Here's how the part is built. I have some questions about the finished solid (model axes, mm). A direction names the side the tool comes from. Round coordinates to 2 decimals unless told otherwise and drop trailing zeros. Loops run counter-clockwise (first coordinate to the right, second up) from the corner with the lowest first, then second, coordinate; pieces in that order, holes last. Notation, with made-up numbers: M 60.25,-35.75 L 90.25,-35.75 A14 ccw 90.25,-10.75 Z; hole C 34.5,71.25 d1. An arc over 180 degrees is marked long. Answer as a JSON object with one key per item and string values.
from build123d import *

# Parameters (mm, degrees)
F0_W          = 28.448
F0_H          = 31.75
F1_DEPTH      = 73.406
F3_DEPTH      = 7.874
F4_W          = 6.35
F4_H          = 28.448
F5_DEPTH      = 4.826
F6_DEPTH      = 4.826
F6_DEPTH_BACK = 20.574


# Not quite as in the source:
# - a pattern or mirror of a feature is missing from the dataset's text; its kind, count and spacing are read off the source's solid


with BuildPart() as f1:
    # F0 (on Right) → F1 (new body)
    with BuildSketch(Plane.YZ):
        Rectangle(F0_W, F0_H)
    extrude(amount=F1_DEPTH)

    # F2 (on Front) → F3 (join, symmetric)
    with BuildSketch(Plane.XZ):
        Polygon((0, 15.875), (73.406, 15.875), (76.2, 15.875), (104.648, 44.323), (0, 44.323), align=None)
        with BuildLine():
            ThreePointArc((30.226, 24.511), (24.638, 30.099), (30.226, 35.687))
            Line((30.226, 35.687), (54.102, 35.687))
            ThreePointArc((54.102, 35.687), (58.0533126933, 34.0503126933), (59.69, 30.099))
            ThreePointArc((59.69, 30.099), (58.0533126933, 26.1476873067), (54.102, 24.511))
            Line((54.102, 24.511), (30.226, 24.511))
        make_face(mode=Mode.SUBTRACT)
        Polygon((104.648, -44.323), (76.2, -15.875), (73.406, -15.875), (0, -15.875), (0, -44.323), align=None)
        with BuildLine():
            ThreePointArc((30.226, -35.687), (24.638, -30.099), (30.226, -24.511))
            Line((30.226, -24.511), (54.102, -24.511))
            ThreePointArc((54.102, -24.511), (58.0533126933, -26.1476873067), (59.69, -30.099))
            ThreePointArc((59.69, -30.099), (58.0533126933, -34.0503126933), (54.102, -35.687))
            Line((54.102, -35.687), (30.226, -35.687))
        make_face(mode=Mode.SUBTRACT)
    extrude(amount=F3_DEPTH, both=True)

    # F4 (on face) → F5 (cut)
    with BuildSketch(Plane.XZ.offset(7.874)):
        with Locations((3.175, 30.099)):
            Rectangle(F4_W, F4_H)
    f5 = extrude(amount=-F5_DEPTH, mode=Mode.SUBTRACT)

    # F5_copies: F5 across plane
    add(f5.mirror(Plane(origin=(0, 0, 0), x_dir=(-1, 0, 0), z_dir=(0, 0, -1))), mode=Mode.SUBTRACT)

    # F4 (on face) → F6 (join, two sides)
    with BuildSketch(Plane.XZ.offset(7.874)) as f6_sk:
        Polygon((104.648, 44.323), (69.596, 44.323), (69.596, 26.797), (87.122, 26.797), align=None)
    f6 = extrude(amount=F6_DEPTH) + extrude(f6_sk.sketch, amount=-F6_DEPTH_BACK)

    # F6_copies: F6 across plane
    add(f6.mirror(Plane(origin=(0, 0, 0), x_dir=(-1, 0, 0), z_dir=(0, 0, -1))))


solid = f1.part
Item 1: I want a section at D-D on z = 33. List the corners of the cut face in (x, y) for me (3 decimals).
Solution:
{"outline": "M 0,-3.048 L 6.35,-3.048 L 6.35,-7.874 L 25.45,-7.874 L 25.45,7.874 L 0,7.874 Z; M 58.878,-7.874 L 69.596,-7.874 L 69.596,-12.7 L 93.325,-12.7 L 93.325,12.7 L 69.596,12.7 L 69.596,7.874 L 58.878,7.874 Z"}
Item 2: We'd pull the mould along X, two halves only. Please class faces 5 (the face through (69.596, -10, -36)), 6 (the face through (42, 0, 35.687)), 7 (the face through (75, 0, -15.875)), 8 (the face through (73.406, 0, 0)): +X half, -X half, draft (parallel to the pull), parting line (faces both ways), or undercut.
Solution:
{"face 5": "-X half", "face 6": "undercut", "face 7": "draft", "face 8": "+X half"}
Item 3: I want a section at A-A on x = 39. List the corners of the cut face in (y, z) for me (3 decimals), plus the area to 3 significant figures.
Solution:
{"outline": "M -14.224,-15.875 L -7.874,-15.875 L -7.874,-24.511 L 7.874,-24.511 L 7.874,-15.875 L 14.224,-15.875 L 14.224,15.875 L 7.874,15.875 L 7.874,24.511 L -7.874,24.511 L -7.874,15.875 L -14.224,15.875 Z; M -7.874,-44.323 L 7.874,-44.323 L 7.874,-35.687 L -7.874,-35.687 Z; M -7.874,35.687 L 7.874,35.687 L 7.874,44.323 L -7.874,44.323 Z", "area": "1,450 mm2"}
Item 4: I want a section at C-C on x = 97. List the corners of the cut face in (y, z) for me (3 decimals).
Solution:
{"outline": "M -12.7,-44.323 L 12.7,-44.323 L 12.7,-36.675 L -12.7,-36.675 Z; M -12.7,36.675 L 12.7,36.675 L 12.7,44.323 L -12.7,44.323 Z"}
Item 5: For P1, Ø14, axis at x = 25, z = -30.5, coming from the +Y side; P2, Ø2.5, axis at y = -11.5, z = -35, coming from the -X side; P3, Ø23, axis at x = 45, z = 29.5, coming from the -Y side, each with a flat end and sliding along its axis, tell me the tip position at first contact or that it passes through.
Solution:
{"P1": "stops at y = 7.87", "P2": "stops at x = 69.6", "P3": "stops at y = -7.87"}
Item 6: I want a section at B-B on y = 4.75. List the corners of the cut face in (x, z) for me (3 decimals).
Solution:
{"outline": "M 0,-44.323 L 104.648,-44.323 L 76.2,-15.875 L 73.406,-15.875 L 73.406,15.875 L 76.2,15.875 L 104.648,44.323 L 0,44.323 Z; hole M 30.226,-35.687 L 54.102,-35.687 A5.588 ccw 54.102,-24.511 L 30.226,-24.511 A5.588 ccw Z; hole M 30.226,24.511 L 54.102,24.511 A5.588 ccw 54.102,35.687 L 30.226,35.687 A5.588 ccw Z"}
Item 7: For faces 1 (the face through (83, 12.7, 36)), 2 (the face through (93.386, 0.178, -33.061)), 3 (the face through (83, -12.7, -36)), 4 (the face through (42, 0, -35.687)), which set-ups out of +Z, -Z, +X, -X, +Y, -Y let a thin tool reach every point of the face, with its end or its side?
Solution:
{"face 1": "+Z, +X, -X, +Y", "face 2": "+X, +Y, -Y", "face 3": "-Z, +X, -X, -Y", "face 4": "+Y, -Y"}
Item 8: If I drill on L1, parallel to Z at x = 37, y = 5.5; L2, parallel to Z at x = 75, y = 7.25 (3 decimals); L3, parallel to Z at x = 80, y = 11, over which ranges is the centre line in solid material (lowest first)? Write a range as from..to.
Solution:
{"L1": "z = -44.32..-35.69, -24.51..24.51, 35.69..44.32", "L2": "z = -44.323..-15.875, 15.875..44.323", "L3": "z = -44.32..-26.8, 26.8..44.32"}
